Part model, mm, in its own coordinate system. A direction names the side the tool comes from. Give positions to 0.01 mm unless a question says otherwise; leave off trailing zeros. Order: outer loops, then holes, each group sorted by start corner. A loop starts at its lowest first (then second) coordinate and runs counter-clockwise, first axis right, second up. Notation, with made-up numbers: M 56.25,57.25 L 95.25,57.25 A22 cw 95.25,79.25 Z; hole C -26,-23.5 d1. An arc over 180 degrees is marked long. Answer as a JSON object with one key per item and string values.
from build123d import *

# Parameters (mm, degrees)
SKETCH1_R           = 217.5
BOSS_EXTRUDE1_DEPTH = 30
SKETCH2_R           = 75
BOSS_EXTRUDE2_DEPTH = 2.5
SKETCH3_R           = 70
BOSS_EXTRUDE3_DEPTH = 57.5
SKETCH12_R          = 22.5
CUT_EXTRUDE2_DEPTH  = 30
FILLET2_R           = 10
SCALE2_SCALE        = 0.1
SKETCH14_R          = 4.45
CUT_EXTRUDE3_DEPTH  = 4.5


with BuildPart() as part:
    # Sketch1 → Boss-Extrude1 (new body)
    with BuildSketch(Plane.XY):
        Circle(SKETCH1_R)
    extrude(amount=BOSS_EXTRUDE1_DEPTH)

    # Sketch2 → Boss-Extrude2 (add)
    with BuildSketch(Plane.XY.offset(30)):
        Circle(SKETCH2_R)
    extrude(amount=BOSS_EXTRUDE2_DEPTH)

    # Sketch3 → Boss-Extrude3 (add)
    with BuildSketch(Plane.XY.offset(32.5)):
        Circle(SKETCH3_R)
    extrude(amount=BOSS_EXTRUDE3_DEPTH)

    # Sketch12 → Cut-Extrude2 (cut)
    with BuildSketch(Plane.XY.offset(30)):
        with Locations((0, 155)):
            Circle(SKETCH12_R)
        with Locations((109.601551084, 109.601551084)):
            Circle(SKETCH12_R)
        with Locations((155, 0)):
            Circle(SKETCH12_R)
        with Locations((109.601551084, -109.601551084)):
            Circle(SKETCH12_R)
        with Locations((0, -155)):
            Circle(SKETCH12_R)
        with Locations((-109.601551084, -109.601551084)):
            Circle(SKETCH12_R)
        with Locations((-155, 0)):
            Circle(SKETCH12_R)
        with Locations((-109.601551084, 109.601551084)):
            Circle(SKETCH12_R)
    extrude(amount=-CUT_EXTRUDE2_DEPTH, mode=Mode.SUBTRACT)

    # Fillet2
    fillet2_edges = [part.edges().sort_by_distance(p)[0] for p in [
        (-217.5, 0, 0),
        (-217.5, 0, 30),
    ]]
    fillet(fillet2_edges, radius=FILLET2_R)


with BuildPart() as part_1:
    # Scale2: scaled about (0, 0, 23.418586113)
    add(part.part.scale(SCALE2_SCALE).moved(Location((0, 0, 21.076727502))))

    # Sketch14 → Cut-Extrude3 (cut)
    with BuildSketch(Plane.XY.offset(30.076727502)):
        Circle(SKETCH14_R)
    extrude(amount=-CUT_EXTRUDE3_DEPTH, mode=Mode.SUBTRACT)


solid = part_1.part
1. Cut at C-C on z = 27.75. Give the cut face in (x, y), plus the area to 3 significant figures.
Worked answers:
{"outline": "C 0,0 d14; hole C 0,0 d8.9", "area": "91.7 mm^2"}
2. Which spindle directions (+Z, -Z, +X, -X, +Y, -Y) get a long thin tool onto all of the face, cutting with end or side? Do faces 4 (the flat face through (0, 0, 25.577)), 5 (the cylindrical face through (17.646, 0.676, 22.598)). Say none if no direction does.
Worked answers:
{"face 4": "+Z", "face 5": "+Z, -Z"}
3. Cut at A-A on y = 0. Give the cut face in (x, z), plus the area to 3 significant figures.
Worked answers:
{"outline": "M -21.75,22.08 A1 ccw -20.75,21.08 L -17.75,21.08 L -17.75,24.08 L -20.75,24.08 A1 ccw -21.75,23.08 Z; M -13.25,21.08 L 13.25,21.08 L 13.25,24.08 L 7.5,24.08 L 7.5,24.33 L 7,24.33 L 7,30.08 L 4.45,30.08 L 4.45,25.58 L -4.45,25.58 L -4.45,30.08 L -7,30.08 L -7,24.33 L -7.5,24.33 L -7.5,24.08 L -13.25,24.08 Z; M 17.75,21.08 L 20.75,21.08 A1 ccw 21.75,22.08 L 21.75,23.08 A1 ccw 20.75,24.08 L 17.75,24.08 Z", "area": "147 mm^2"}
4. Cut at D-D on x = 12.5. State how many separate pieces and enclosed holes the cut face has, plus the area to 3 significant figures.
Worked answers:
{"separate pieces": "3", "enclosed holes": "0", "area": "86.1 mm^2"}
5. Pin check, flat tips, straight feed: P1, Ø7, axis at x = -15.5, y = 0, coming from the -Z side; P2, Ø6, axis at x = 15.5, y = 0, coming from the +Z side; P3, Ø4, axis at x = 5, z = 22, coming from the +Y side; P4, Ø2.5, axis at x = 0.5, y = 0.5, coming from the +Z side. Stop position of each tip, or through.
Worked answers:
{"P1": "stops at z = 21.08", "P2": "stops at z = 24.08", "P3": "stops at y = 21.54", "P4": "stops at z = 25.58"}
6. Probe line 1 along Y through (x, z) = (0, 29.1); line 2 along Z through (x, y) = (19, 5); line 3 along X through (y, z) = (-15.5, 22.8). List the from-to ranges inside material, lowest first.
Worked answers:
{"line 1": "y = -7 to -4.45, 4.45 to 7", "line 2": "z = 21.08 to 24.08", "line 3": "x = -15.26 to -2.25, 2.25 to 15.26"}
7. Two-plate mould, pull along X, no slides. Class faces 1 (the flat face through (0, -5, 30.077)), 2 (the cylindrical face through (10.67, -8.73, 22.6)), 3 (the cylindrical face through (6.466, -2.681, 27.161)): +X half, -X half, draft (parallel to the pull), parting line (faces both ways), or undercut.
Worked answers:
{"face 1": "draft", "face 2": "undercut", "face 3": "parting line"}
